Can you work these out from the model? Positions are in its coordinate system, mm. A direction names the side the tool comes from. Coordinates: 2 decimals unless noted, no trailing zeros. Put each result on its own line as item: value. Start each with the question number.
Item 1: For faces 5 (the flat face through (0, 8, -13)), 6 (the cylindrical face through (27.25, 10.36, -4.83)), which set-ups out of +Z, -Z, +X, -X, +Y, -Y let a thin tool reach every point of the face, with its end or its side?
Item 2: If we section it at A-A on z = -6.5: State how many separate pieces and enclosed holes the cut face has, plus the area to 3 significant figures.
Item 3: Will these pins go through, and if not, where does the flat tip stop? P1, Ø5, axis at x = 116, y = 8.5, coming from the -Z side; P2, Ø5.5, axis at x = 25.4, y = 7.94, coming from the +Z side; P3, Ø1.5, axis at y = 10, z = -25, coming from the -X side.
Item 4: We'd pull the mould along Y, two halves only. Please class faces 1 (the flat face through (150, 0, -14)), 2 (the cylindrical face through (276.378, 8.334, -4.829)), 3 (the flat face through (150.311, 11.166, -25.346)), 4 (the flat face through (304.8, 8, -13)): pulls with the +Y half, pulls with the -Y half, needs draft (parallel to the pull), parting line crosses it, or undercut.
Item 5: Please list where these lines run through material, in increasing order: L1, parallel to Y at x = 279.4, z = -7 (1 decimal); L2, parallel to X at y = 2.75, z = -9.5; L3, parallel to X at y = 9.25, z = -8. Write a range as from..to.
Autodesk Inventor part; units mm, degrees
ref_plane "YZ Plane" through (0, 0, 0) normal (1, 0, 0) x (0, 1, 0)
ref_plane "XZ Plane" through (0, 0, 0) normal (0, 1, 0) x (-1, 0, 0)
ref_plane "XY Plane" through (0, 0, 0) normal (0, 0, 1) x (1, 0, 0)
sketch "Sketch1" plane through (0, 0, 0) normal (1, 0, 0) x (0, 1, 0)
  line L0 (0, 0) -> (30.1625, 0)
  line L1 (30.1625, 0) -> (30.1625, -6.35)
  line L2 (30.1625, -6.35) -> (6.35, -30.1625)
  line L3 (6.35, -30.1625) -> (0, -30.1625)
  line L4 (0, -30.1625) -> (0, 0)
  line L5 (15.875, 0) -> (15.875, -20.6375)
  point P0 (15.0812, 0)
  dimension "d0" = 30.1625
  dimension "d1" = 6.35
  dimension "d16" = 15.875
extrude "Extrusion1" add sketch "Sketch1" along normal blind 304.8 contours L0 L5 L2 L3 L4
sketch "Sketch2" plane through (0, 0, 0) normal (0, 0, 1) x (1, 0, 0)
  line L0 (0, 15.875) -> (0, 0)
  line L1 (0, 0) -> (304.8, 0)
  point P0 (25.4, 7.9375)
  point P1 (152.4, 7.9375)
  point P2 (279.4, 7.9375)
  point P3 (152.4, 0)
  dimension "d4" = 25.4
  dimension "d5" = 7.9375
  dimension "d6" = 25.4
hole "Hole1" at (25.4, 7.9375, 0) at (152.4, 7.9375, 0) at (279.4, 7.9375, 0) direction (0, 0, -1) diameter 6.096 depth 9.525 tip angle 118
fillet "Fillet1" radius 3.175 11 edges at (152.4, 6.35, -30.1625) (152.4, 0, -30.1625) (0, 11.1125, -25.4) (0, 3.175, -30.1625) (0, 0, -15.0812) (304.8, 3.175, -30.1625) (304.8, 0, -15.0812) (304.8, 11.1125, -25.4) (152.4, 15.875, -20.6375) (304.8, 15.875, -10.3188) (0, 15.875, -10.3188)
properties part number "3DPRINT,BELT,GUARD" material "ABS Plastic"
Solutions:
1. face 5: +Z, -Z, -X, +Y, -Y
1. face 6: +Z
2. separate pieces: 1
2. enclosed holes: 3
2. area: 4,740 mm^2
3. P1: z = -30.01
3. P2: z = -9.7
3. P3: x = 0.3
4. face 1: pulls with the -Y half
4. face 2: undercut
4. face 3: pulls with the +Y half
4. face 4: needs draft
5. L1: 0..4.9, 11..15.9
5. L2: 0.03..304.77
5. L3: 0..22.65, 28.15..149.65, 155.15..276.65, 282.15..304.8
